Source: CAD feature listing. Evaluate the final solid. Frame: model axes, mm. A direction names the side the tool comes from. Coordinates: 2 decimals unless noted, no trailing zeros. Loops run counter-clockwise (first coordinate to the right, second up) from the corner with the lowest first, then second, coordinate; pieces in that order, holes last. Notation, with made-up numbers: M -0.75,-28.5 L 47.25,-28.5 A30 cw 47.25,5.5 Z; hole C -30.75,-5 d2. An arc over 180 degrees is marked long. One line per question, with ' | ' between items. Start each with the question number.
1. Section query A-A, the plane z = 0. Output: boundary loops of the cut face in (x, y), and give its area (3 significant figures).
2. Ray query, probe 1 along Y at (x, z) = (-0.15, 0); probe 2 along Z at (x, y) = (-7.5, 0). Return the intervals inside material, ascending.
3. Pin query (flat end, axial travel): P1, Ø4, axis at x = -4.5, z = -6.5, coming from the -Y side; P2, Ø3, axis at x = -4, y = -3.5, coming from the -Z side; P3, Ø4, axis at x = -4, y = -18.5, coming from the -Z side. Return the tip coordinate at first contact, or that it passes through.
4. Access query for faces 4 (the flat face through (-6.8, 0, 0)), 5 (the flat face through (-7.6, 5, -28.3)), 6 (the flat face through (-0.8, 0, -7)). Directions: +Z, -Z, +X, -X, +Y, -Y. A direction counts if a zero-diameter tool reaches every point of the face in a straight line with its end or side. Return the directions, or none.
5. Section query C-C, the plane x = -3.5. Output: boundary loops of the cut face in (y, z).
6. Mould query, pull axis Y, two halves, no side actions, for faces 1 (the cylindrical face through (-7.45, -6.18, 27.82)), 2 (the cylindrical face through (-3.853, 32.907, -10.363)), 3 (the flat face through (0, -5, -28.3)). Classes: pulls with the +Y half, pulls with the -Y half, needs draft (parallel to the pull), parting line crosses it, or undercut.
```python
from build123d import *

# Parameters (mm, degrees)
FILLET1_R = 0.5


with BuildPart() as part:
    # Sketch3 → Revolve1 (revolve)
    with BuildSketch(Plane.XY):
        Polygon((-7.6, 28.5), (-6.8, 28.5), (-6.8, 0), (-0.8, 0), (0, 0), (0, 6.35), (-0.8, 6.35), (-0.8, 28.5), (0, 28.5), (0, 34.5), (-7.6, 34.5), align=None)
    revolve(axis=Axis((-0.8, 0, 0), (-1, 0, 0)))

    # Fillet1
    fillet1_edges = [part.edges().sort_by_distance(p)[0] for p in [
        (-6.8, -28.5, 0),
        (-0.8, -28.5, 0),
    ]]
    fillet(fillet1_edges, radius=FILLET1_R)


solid = part.part
```
Taken from the geometry:
1) outline: M -7.6,-34.5 L 0,-34.5 L 0,-28.5 L -0.3,-28.5 A0.5 cw -0.8,-28 L -0.8,-6.35 L 0,-6.35 L 0,6.35 L -0.8,6.35 L -0.8,28 A0.5 cw -0.3,28.5 L 0,28.5 L 0,34.5 L -7.6,34.5 L -7.6,28.5 L -7.3,28.5 A0.5 cw -6.8,28 L -6.8,-28 A0.5 cw -7.3,-28.5 L -7.6,-28.5 Z | area: 444 mm^2
2) probe 1: -34.5 to -28.5, -6.35 to 6.35, 28.5 to 34.5 | probe 2: -34.5 to -28.5, 28.5 to 34.5
3) P1: y = -34.21 | P2: z = -34.44 | P3: z = -30.3
4) face 4: -X | face 5: +Z, -Z, -X, +Y, -Y | face 6: +X
5) outline: C 0,0 d69
6) face 1: undercut | face 2: parting line crosses it | face 3: needs draft
